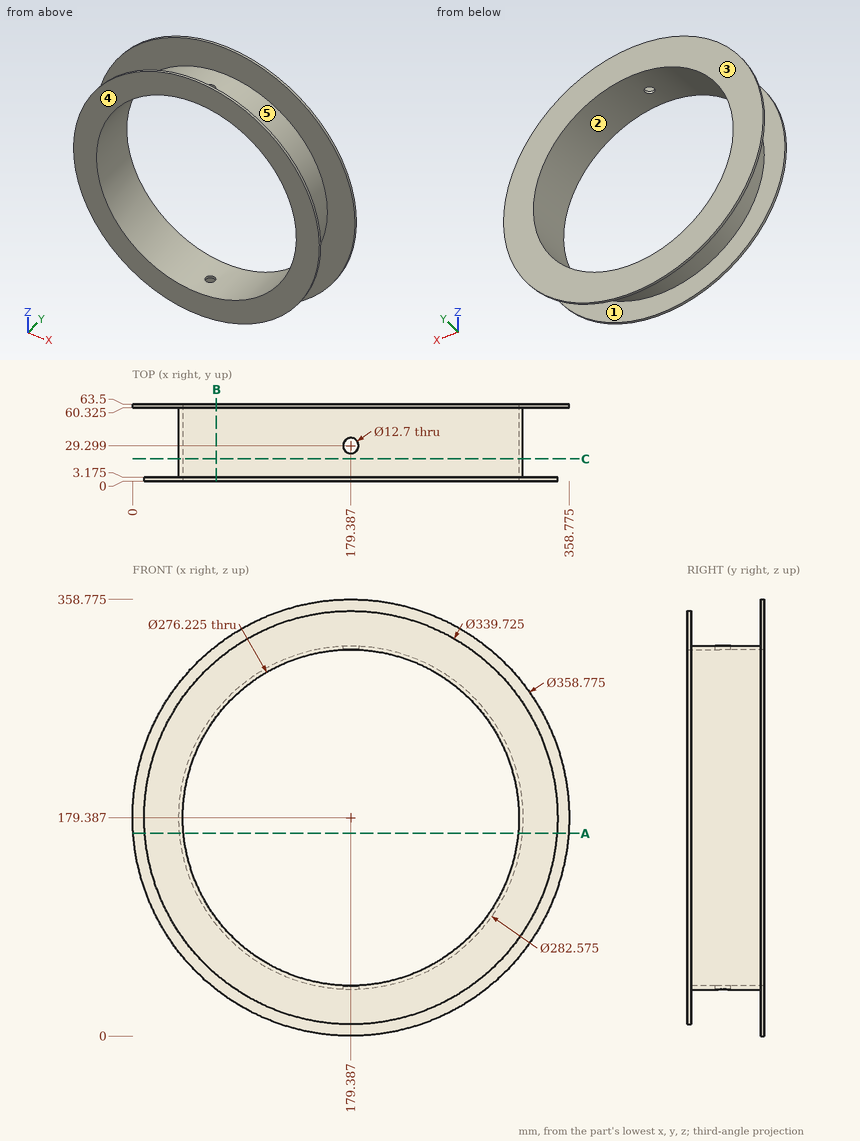
For this review, use the dimensioned drawing (mm, ordinates from the lowest corner) and the shaded views. A direction names the side the tool comes from. Coordinates: 2 decimals unless noted, no trailing zeros. Loops run counter-clockwise (first coordinate to the right, second up) from the corner with the lowest first, then second, coordinate; pieces in that order, holes last. Notation, with made-up numbers: (-16.75, 49.25) - (29.25, 49.25) arc R11 ccw to (29.25, 68.25) - close; hole circle Ø10 at (37.25, 17). An arc over 180 degrees is marked (long way). Use one line per item in the form item = value. Start each with the question number.
1) For pin 1 (12 mm diameter, centred on y = 14, z = 306.5, fed in from +X) (1 decimal); pin 2 (3 mm diameter, centred on y = 31.5, z = 108.5, fed in from -X); pin 3 (8 mm diameter, centred on y = 10.5, z = 177, fed in from +X) (1 decimal), all flat-tipped, find the tip position at first contact; note any pin that passes through.
2) Draft analysis for pull direction Y (two halves, no side actions). For the marked faces 3, 4 and 5, state which applies: released by +Y, released by -Y, zero draft, split by the parting line, or undercut.
3) For the marked faces 1 and 2, list the 3-axis set-ups (+Z, -Z, +X, -X, +Y, -Y) from which the entire face can be reached by the end or side of a thin tool; tool diameter is ignored.
4) Take a section at B-B (x = 69). State the section outline as (y, z) points (1 decimal).
5) Take a section at A-A (z = 166.5). State the section outline as (x, y) points (1 decimal).
6) To check wall thickness, follow probe 1 along Y at (x, z) = (185.5, 22.5) (1 decimal); probe 2 along X at (y, z) = (50, 284.5) (1 decimal); probe 3 along Z at (x, y) = (108.5, 33) (1 decimal). State the ranges of each line that lie inside material, in increasing order. Write a range as from..to.
7) Take a section at C-C (y = 18.5). State the section outline as (x, z) points (1 decimal), plus the area to 3 significant figures.
From the geometry:
q1.pin_1 = 252.1
q1.pin_2 = 56.31
q1.pin_3 = 320.7
q2.face_3 = released by +Y
q2.face_4 = released by -Y
q2.face_5 = undercut
q3.face_1 = none
q3.face_2 = +Y, -Y
q4.outline = (0, 50.3) - (3.2, 50.3) - (3.2, 91.2) - (60.3, 91.2) - (60.3, 38) - (63.5, 38) - (63.5, 96.4) - (0, 96.4) - close; (0, 262.4) - (63.5, 262.4) - (63.5, 320.8) - (60.3, 320.8) - (60.3, 267.6) - (3.2, 267.6) - (3.2, 308.5) - (0, 308.5) - close
q5.outline = (0.5, 60.3) - (38.7, 60.3) - (38.7, 3.2) - (10, 3.2) - (10, 0) - (41.9, 0) - (41.9, 63.5) - (0.5, 63.5) - close; (316.9, 0) - (348.8, 0) - (348.8, 3.2) - (320.1, 3.2) - (320.1, 60.3) - (358.3, 60.3) - (358.3, 63.5) - (316.9, 63.5) - close
q6.probe_1 = 0..3.2, 60.3..63.5
q6.probe_2 = 85..89.8, 269..273.8
q6.probe_3 = 57.2..60.9, 297.9..301.6
q7.outline = circle Ø282.6 at (179.4, 179.4); hole circle Ø276.2 at (179.4, 179.4)
q7.area = 2,790 mm2
